The model under review builds one solid part; all positions refer to its coordinate system, in mm. Coordinates: 2 decimals unless noted, no trailing zeros. Loops run counter-clockwise (first coordinate to the right, second up) from the corner with the lowest first, then second, coordinate; pieces in that order, holes last. Notation, with made-up numbers: (82, 48) - (118, 48) arc R35 cw to (118, 85) - close; hole circle Ø8 at (85.5, 62). An arc over 180 degrees is marked (long way). Use a Markdown table: item, result. Add a question column.
1) To check wall thickness, follow L1, parallel to Z at x = -60.25, y = 15.5; L2, parallel to Y at x = -61.4, z = 72; L3, parallel to Z at x = -60.5, y = 13. State the ranges of each line that lie inside material, in increasing order. Write a range as [from, to].
2) Add section B-B, the plane y = 16. Give the boundary of the cut face in (x, z), and give its area (3 significant figures).
3) The part is to be moulded in two halves that separate along Y. For faces 1 (the flat face through (-60, 30, 88)), 2 (the cylindrical face through (-60.99, 18.7, 74.95)), say which applies: pulls with the +Y half, pulls with the -Y half, needs draft (parallel to the pull), parting line crosses it, or undercut.
4) Add section A-A, the plane z = 112. Give the boundary of the cut face in (x, y).
```python
from build123d import *

# Parameters (mm, degrees)
SKETCH2_W             = 182
SKETCH2_H             = 60
BOSS_EXTRUDE1_DEPTH   = 2
F_8_0MM_DOWEL_HOLE2_D = 8


with BuildPart() as part:
    # Sketch2 → Boss-Extrude1 (new body)
    with BuildSketch(Plane.ZY.offset(60)):
        with Locations((89, 30)):
            Rectangle(SKETCH2_W, SKETCH2_H)
    extrude(amount=BOSS_EXTRUDE1_DEPTH)

    # Ø8.0mm Dowel Hole2 (through all)
    with Locations(Plane.ZY.offset(62)):
        with Locations((112, 16), (72, 16)):
            Hole(F_8_0MM_DOWEL_HOLE2_D / 2)


solid = part.part
```
From the geometry:
| question | item | result |
|---|---|---|
| 1 | L1 | z = [-2, 68.03], [75.97, 108.03], [115.97, 180] |
| 1 | L2 | y = [0, 12], [20, 60] |
| 1 | L3 | z = [-2, 69.35], [74.65, 109.35], [114.65, 180] |
| 2 | outline | (-62, -2) - (-60, -2) - (-60, 68) - (-62, 68) - close; (-62, 76) - (-60, 76) - (-60, 108) - (-62, 108) - close; (-62, 116) - (-60, 116) - (-60, 180) - (-62, 180) - close |
| 2 | area | 332 mm^2 |
| 3 | face 1 | needs draft |
| 3 | face 2 | undercut |
| 4 | outline | (-62, 0) - (-60, 0) - (-60, 12) - (-62, 12) - close; (-62, 20) - (-60, 20) - (-60, 60) - (-62, 60) - close |
